Geometry: see drawing. Coordinates: mm, zero at the bounding-box minimum. Give positions to 0.01 mm unless a question says otherwise; leave off trailing zeros. Write each loop counter-clockwise with the first axis right and the second up, starting at its lowest first coordinate (ties: lowest second). Pieces come first, ordered by that corner, then holes. Notation, with made-up numbers: M 8,45 L 43,45 A32 cw 43,80 Z; hole C 84.25,74 d2. An arc over 180 degrees is marked long. Use a Markdown table: item, result. Add a question column.
1) Pin query (flat end, axial travel): pin 1 (3.5 mm diameter, centred on x = 167, z = 98, fed in from +Y). Return the tip coordinate at first contact, or that it passes through.
2) Section B-B on x = 143. Return the cut outline in (y, z), then the cut area to 3 significant figures.
3) Line query: line 1 (Z direction, x = 167.5, y = 3.75); line 2 (X direction, y = 2.75, z = 10); line 3 (X direction, y = 7.5, z = 56.5). Output: solid intervals per line, ascending.
4) Section A-A on y = 4.75. Return the cut outline in (x, z), then the cut area to 3 significant figures.
5) Section C-C on z = 37.5. Return the cut outline in (x, y), then the cut area to 3 significant figures.
6) Section D-D on x = 167. Return the cut outline in (y, z), then the cut area to 3 significant figures.
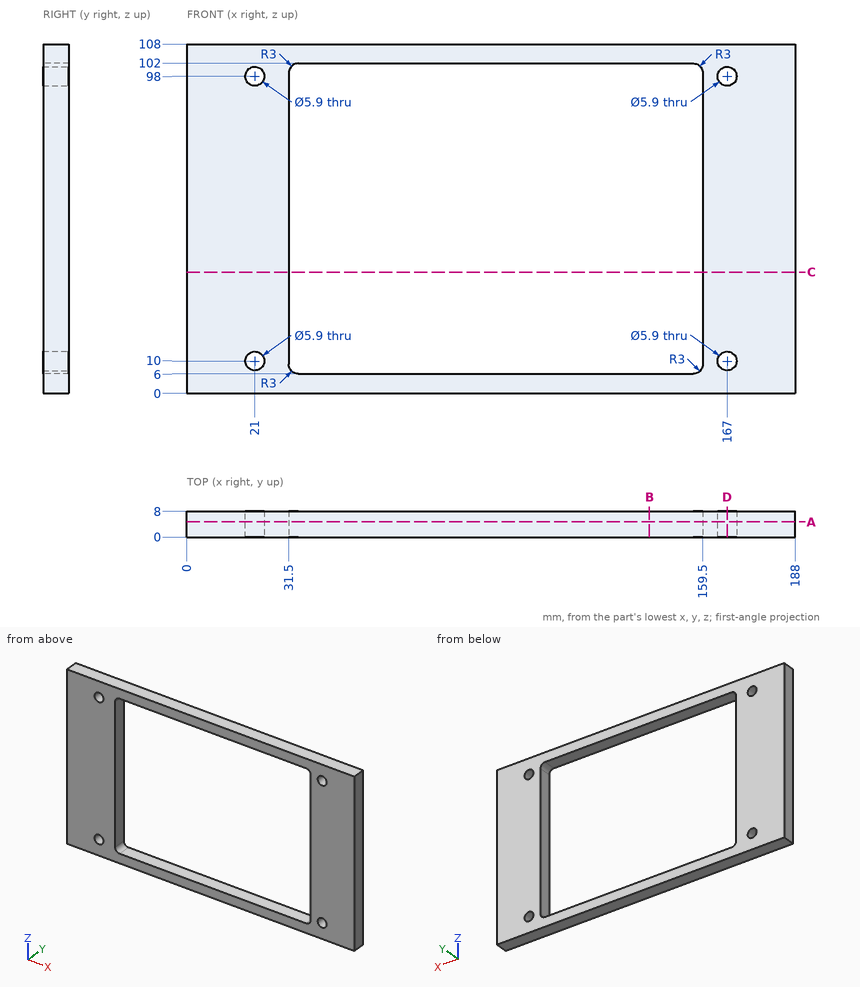
Found:
| question | item | result |
|---|---|---|
| 1 | pin 1 | through |
| 2 | outline | M 0,0 L 8,0 L 8,6 L 0,6 Z; M 0,102 L 8,102 L 8,108 L 0,108 Z |
| 2 | area | 96.0 mm² |
| 3 | line 1 | 0 to 7.09, 12.91 to 95.09, 100.91 to 108 |
| 3 | line 2 | 0 to 18.05, 23.95 to 31.5, 159.5 to 164.05, 169.95 to 188 |
| 3 | line 3 | 0 to 31.5, 159.5 to 188 |
| 4 | outline | M 0,0 L 188,0 L 188,108 L 0,108 Z; hole C 21,10 d5.9; hole C 21,98 d5.9; hole M 31.5,9 A3 ccw 34.5,6 L 156.5,6 A3 ccw 159.5,9 L 159.5,99 A3 ccw 156.5,102 L 34.5,102 A3 ccw 31.5,99 Z; hole C 167,10 d5.9; hole C 167,98 d5.9 |
| 4 | area | 7,910 mm² |
| 5 | outline | M 0,0 L 31.5,0 L 31.5,8 L 0,8 Z; M 159.5,0 L 188,0 L 188,8 L 159.5,8 Z |
| 5 | area | 480 mm² |
| 6 | outline | M 0,0 L 8,0 L 8,7.05 L 0,7.05 Z; M 0,12.95 L 8,12.95 L 8,95.05 L 0,95.05 Z; M 0,100.95 L 8,100.95 L 8,108 L 0,108 Z |
| 6 | area | 770 mm² |
